```python
from build123d import *

# Parameters (mm, degrees)
F0_R      = 9
F1_DEPTH  = 140
F2_DEPTH  = 100
F4_DEPTH  = 10.751
F5_COUNT  = 3
F0_R_2    = 2.25
F6_DEPTH  = 4
F7_START  = 46
F7_DEPTH  = 4
F8_START  = 62
F0_R_3    = 7.5
F8_DEPTH  = 3
F10_DEPTH = 25


# Not quite as in the source:
# - a feature names something its author has since deleted; it is built from what else it names


with BuildPart() as f1:
    # F0 (on Top) → F1 (new body)
    with BuildSketch(Plane.XY):
        with BuildLine():
            ThreePointArc((-3, -9.5393920142), (-2.2464281062, -9.744411771), (-1.4791551643, -9.89))
            ThreePointArc((-1.4791551643, -9.89), (0, -10), (1.4791551643, -9.89))
            ThreePointArc((1.4791551643, -9.89), (2.2464281062, -9.744411771), (3, -9.5393920142))
            ThreePointArc((3, -9.5393920142), (8.0622577483, -5.9160797831), (10, 0))
            ThreePointArc((10, 0), (7.3314391493, 6.8007352544), (0.75, 9.9718353376))
            ThreePointArc((0.75, 9.9718353376), (0, 10), (-0.75, 9.9718353376))
            ThreePointArc((-0.75, 9.9718353376), (-9.9341644436, 1.1455901566), (-3, -9.5393920142))
        make_face()
        Circle(F0_R, mode=Mode.SUBTRACT)
    extrude(amount=F1_DEPTH)

    # F0 (on Top) → F2 (join)
    with BuildSketch(Plane.XY):
        with BuildLine():
            Line((-0.75, 34.9718353376), (-0.75, 9.9718353376))
            ThreePointArc((-0.75, 9.9718353376), (0, 10), (0.75, 9.9718353376))
            Line((0.75, 9.9718353376), (0.75, 34.9718353376))
            Line((0.75, 34.9718353376), (-0.75, 34.9718353376))
        make_face()
    extrude(amount=F2_DEPTH)

    # F3 (on face) → F4 (cut, through all)
    with BuildSketch(Plane.YZ.offset(0.75)):
        with BuildLine():
            Line((9.9718353376, 100), (9.9718353376, 75))
            Line((9.9718353376, 75), (9.9718353376, 69.1647440576))
            add(Edge.make_bspline(
                [(9.9718353376, 69.1647440576), (10.1832449594, 66.2204140215), (12.0836351221, 52.2918027042), (20.9708053433, 36.8272021249), (33.801245613, 23.6414831262), (34.7842815391, 13.599508776), (34.9718353376, 7.702038365)],
                knots=[0.0899218527, 0.0899218527, 0.0899218527, 0.0899218527, 0.2371904705, 0.3995520788, 0.5544857931, 0.7015059428, 0.7015059428, 0.7015059428, 0.7015059428], degree=3))
            Line((34.9718353376, 7.702038365), (34.9718353376, 100))
            Line((34.9718353376, 100), (9.9718353376, 100))
        make_face()
    extrude(amount=-F4_DEPTH, mode=Mode.SUBTRACT)


with BuildPart() as f5_1:
    # F5: instance of F1
    add(f1.part.rotate(Axis((0, 0, 0), (0, 0, 1)), 1 * 360 / F5_COUNT))


with BuildPart() as f5_2:
    # F5: instance of F1
    add(f1.part.rotate(Axis((0, 0, 0), (0, 0, 1)), 2 * 360 / F5_COUNT))


with BuildPart() as f1_1:
    add(f1.part)

    add(f5_1.part)  # F6 merges F5_1

    add(f5_2.part)  # F6 merges F5_2
    # F0 (on Top) → F6 (join)
    with BuildSketch(Plane.XY):
        with BuildLine():
            ThreePointArc((1.4791551643, -9.89), (0, -10), (-1.4791551643, -9.89))
            ThreePointArc((-1.4791551643, -9.89), (-2.592051841, -10.9896135416), (-3, -12.5))
            ThreePointArc((-3, -12.5), (0, -15.5), (3, -12.5))
            ThreePointArc((3, -12.5), (2.592051841, -10.9896135416), (1.4791551643, -9.89))
        make_face()
        with Locations((0, -12.5)):
            Circle(F0_R_2, mode=Mode.SUBTRACT)
        with BuildLine():
            ThreePointArc((-3, -12.5), (-2.592051841, -10.9896135416), (-1.4791551643, -9.89))
            ThreePointArc((-1.4791551643, -9.89), (-2.2464281062, -9.744411771), (-3, -9.5393920142))
            Line((-3, -9.5393920142), (-3, -12.5))
        make_face()
        with BuildLine():
            ThreePointArc((3, -9.5393920142), (2.2464281062, -9.744411771), (1.4791551643, -9.89))
            ThreePointArc((1.4791551643, -9.89), (2.592051841, -10.9896135416), (3, -12.5))
            Line((3, -12.5), (3, -9.5393920142))
        make_face()
    extrude(amount=F6_DEPTH)

    # F0 (on Top) → F7 (join)
    with BuildSketch(Plane.XY.offset(F7_START)):
        with BuildLine():
            ThreePointArc((1.4791551643, -9.89), (0, -10), (-1.4791551643, -9.89))
            ThreePointArc((-1.4791551643, -9.89), (-2.592051841, -10.9896135416), (-3, -12.5))
            ThreePointArc((-3, -12.5), (0, -15.5), (3, -12.5))
            ThreePointArc((3, -12.5), (2.592051841, -10.9896135416), (1.4791551643, -9.89))
        make_face()
        with Locations((0, -12.5)):
            Circle(F0_R_2, mode=Mode.SUBTRACT)
        with BuildLine():
            ThreePointArc((-3, -12.5), (-2.592051841, -10.9896135416), (-1.4791551643, -9.89))
            ThreePointArc((-1.4791551643, -9.89), (-2.2464281062, -9.744411771), (-3, -9.5393920142))
            Line((-3, -9.5393920142), (-3, -12.5))
        make_face()
        with BuildLine():
            ThreePointArc((3, -9.5393920142), (2.2464281062, -9.744411771), (1.4791551643, -9.89))
            ThreePointArc((1.4791551643, -9.89), (2.592051841, -10.9896135416), (3, -12.5))
            Line((3, -12.5), (3, -9.5393920142))
        make_face()
    extrude(amount=F7_DEPTH)

    # F0 (on Top) → F8 (join)
    with BuildSketch(Plane.XY.offset(F8_START)):
        Circle(F0_R)
        Circle(F0_R_3, mode=Mode.SUBTRACT)
    extrude(amount=F8_DEPTH)

    # F9 (on Front) → F10 (cut)
    with BuildSketch(Plane.XZ):
        with BuildLine():
            ThreePointArc((2.25, 115), (-1.5909902577, 116.5909902577), (0, 112.75))
            ThreePointArc((0, 112.75), (1.5909902577, 113.4090097423), (2.25, 115))
        make_face()
        with BuildLine():
            ThreePointArc((2.25, 103), (1.5909902577, 104.5909902577), (0, 105.25))
            ThreePointArc((0, 105.25), (-1.5909902577, 101.4090097423), (2.25, 103))
        make_face()
    extrude(amount=-F10_DEPTH, mode=Mode.SUBTRACT)


solid = f1_1.part
```
Could you check a few things on this model? Use its own coordinates, in mm. A direction names the side the tool comes from. Coordinates: 2 decimals unless noted, no trailing zeros. Write each loop counter-clockwise with the first axis right and the second up, starting at its lowest first coordinate (ties: lowest second). Pieces come first, ordered by that corner, then holes. Notation, with made-up numbers: (43.5, 67.5) -> (66.5, 67.5) arc R17 cw to (66.5, 95.5) -> close; hole circle Ø9 at (77.25, 1). An arc over 180 degrees is marked (long way). Return JSON: item names as keys, results as strings.
(1) We'd pull the mould along X, two halves only. Please class faces 4 (the flat face through (3, -11, 48)), 5 (the flat face through (2, -11, 50)), 6 (the cylindrical face through (1.21, -10.603, 1.972)): +X half, -X half, draft (parallel to the pull), parting line (faces both ways), or undercut.
Numbers:
{"face 4": "+X half", "face 5": "draft", "face 6": "undercut"}
(2) I need wall thicknesses on L1, parallel to Y at x = 0, z = 2.5; L2, parallel to Y at x = 0, z = 49; L3, parallel to X at y = -7, z = 39. Which ranges of each line are inside material? Lowest first, please.
Numbers:
{"L1": "y = -15.5 to -14.75, -10.25 to -9, 9 to 34.97", "L2": "y = -15.5 to -14.75, -10.25 to -9, 9 to 14.67", "L3": "x = -13.62 to -10.62, -7.14 to -5.66, 5.66 to 7.14, 10.62 to 13.62"}
(3) Imagine slicing it at B-B, the plane z = 48. Count the separate pieces of the cut face and the enclosed holes in it, then the cut area to 3 significant figures.
Numbers:
{"separate pieces": "1", "enclosed holes": "2", "area": "96.9 mm2"}
(4) Imagine slicing it at A-A, the plane z = 91. Please give me the cut outline in (x, y).
Numbers:
{"outline": "circle Ø20 at (0, 0); hole circle Ø18 at (0, 0)"}
(5) Which directions (+Z, -Z, +X, -X, +Y, -Y) give clear straight access to the entire face, cutting with the end or side of a thin tool? Please do faces 1 (the cylindrical face through (-1.172, 8.923, 30.566)), 2 (the flat face through (-0.75, 20, 19)), 3 (the flat face through (-3, -11, 2)).
Numbers:
{"face 1": "-Z", "face 2": "+Z, -Z, -X, +Y", "face 3": "+Z, -Z, -Y"}
(6) I'm going to push flat-ended pins straight in: pin 1 (1.5 mm diameter, centred on y = -10.5, z = 2.5, fed in from +X); pin 2 (5 mm diameter, centred on y = 8.5, z = 50.5, fed in from +X); pin 3 (7 mm diameter, centred on x = 0, z = 115, fed in from +Y). Where does each tip first touch, or does it pass through?
Numbers:
{"pin 1": "stops at x = 20.99", "pin 2": "stops at x = 8", "pin 3": "stops at y = 10"}
